from build123d import *

# Parameters (mm, degrees)
SKETCH1_W                 = 5
SKETCH1_H                 = 7
BOSS_EXTRUDE1_DEPTH       = 2
BOSS_EXTRUDE3_DEPTH       = 3
SKETCH13_W                = 5
SKETCH13_H                = 4
BOSS_EXTRUDE4_DEPTH       = 7
SKETCH14_W                = 4
SKETCH14_H                = 4
BOSS_EXTRUDE6_DEPTH       = 3
FILLET1_R                 = 2.5
M2_CLEARANCE_HOLE3_REACH  = 20.453
M2_CLEARANCE_HOLE3_BORE_R = 1.2
SKETCH15_W                = 3.5
SKETCH15_H                = 4.5
CUT_EXTRUDE1_DEPTH        = 4
M2_CLEARANCE_HOLE2_D      = 2.4
M2_CLEARANCE_HOLE2_DEPTH  = 4
M2_CLEARANCE_HOLE2_TIP    = 0.721032743
SKETCH22_W                = 4
SKETCH22_H                = 16
CUT_EXTRUDE2_DEPTH        = 3


with BuildPart() as part:
    # Sketch1 → Boss-Extrude1 (new, symmetric)
    with BuildSketch(Plane.XY):
        Rectangle(SKETCH1_W, SKETCH1_H)
    extrude(amount=BOSS_EXTRUDE1_DEPTH, both=True)

    # Sketch9 → Boss-Extrude3 (add)
    with BuildSketch(Plane.XZ.offset(3.5)):
        Polygon((2.5, 2), (6.5, 2), (6.5, -2), (2.5, -2), (-2.5, -2), (-2.5, 2), (-2.5, 14), (2.5, 14), align=None)
    extrude(amount=BOSS_EXTRUDE3_DEPTH)

    # Sketch13 → Boss-Extrude4 (add)
    with BuildSketch(Plane(origin=(0, -3.5, 0), x_dir=(1, 0, 0), z_dir=(0, 1, 0))):
        with Locations((0, -12)):
            Rectangle(SKETCH13_W, SKETCH13_H)
    extrude(amount=BOSS_EXTRUDE4_DEPTH)

    # Sketch14 → Boss-Extrude6 (add)
    with BuildSketch(Plane(origin=(0, -3.5, 0), x_dir=(1, 0, 0), z_dir=(0, 1, 0))):
        with Locations((4.5, -12)):
            Rectangle(SKETCH14_W, SKETCH14_H)
    extrude(amount=-BOSS_EXTRUDE6_DEPTH)

    # Fillet1
    # the kernel refuses this fillet: 2.5 mm, written as the material it adds along each edge
    with BuildSketch(Plane(origin=(2.5, -3.5, 2), x_dir=(0, 0, 1), z_dir=(0, -1, 0))) as fillet1_piece_1:
        with BuildLine():
            CenterArc((FILLET1_R, -FILLET1_R), FILLET1_R, 90, 90)
            Line((0, -FILLET1_R), (0, 0))
            Line((0, 0), (FILLET1_R, 0))
        make_face()
    extrude(amount=3)
    with BuildSketch(Plane(origin=(2.5, -3.5, 10), x_dir=(0, 0, -1), z_dir=(0, -1, 0))) as fillet1_piece_2:
        with BuildLine():
            CenterArc((FILLET1_R, FILLET1_R), FILLET1_R, 180, 90)
            Line((0, FILLET1_R), (0, 0))
            Line((0, 0), (FILLET1_R, 0))
        make_face()
    extrude(amount=3)

    # M2 Clearance Hole3 bore → M2 Clearance Hole3 (cut, up to next)
    with BuildSketch(Plane.XY.offset(14), mode=Mode.PRIVATE) as m2_clearance_hole3_sk1:
        Circle(M2_CLEARANCE_HOLE3_BORE_R)
    m2_clearance_hole3_tool1 = extrude(m2_clearance_hole3_sk1.sketch, amount=-M2_CLEARANCE_HOLE3_REACH, mode=Mode.PRIVATE) & part.part
    add(m2_clearance_hole3_tool1.solids().sort_by_distance((0, 0, 14))[0], mode=Mode.SUBTRACT)

    # Sketch15 → Cut-Extrude1 (cut)
    with BuildSketch(Plane(origin=(0, 0, -2), x_dir=(-1, 0, 0), z_dir=(0, 0, -1))):
        Rectangle(SKETCH15_W, SKETCH15_H)
    extrude(amount=-CUT_EXTRUDE1_DEPTH, mode=Mode.SUBTRACT)

    # M2 Clearance Hole2
    with Locations(Plane(origin=(0, -3.5, 0), x_dir=(1, 0, 0), z_dir=(0, 1, 0))):
        with Locations((4.5, -12), (0, -8), (0, -4), (4.5, 0)):
            Hole(M2_CLEARANCE_HOLE2_D / 2, depth=M2_CLEARANCE_HOLE2_DEPTH)
            with Locations((0, 0, -(M2_CLEARANCE_HOLE2_DEPTH + M2_CLEARANCE_HOLE2_TIP / 2))):  # 118° drill point
                Cone(0, M2_CLEARANCE_HOLE2_D / 2, M2_CLEARANCE_HOLE2_TIP, mode=Mode.SUBTRACT)

    # Sketch22 → Cut-Extrude2 (cut)
    with BuildSketch(Plane(origin=(0, -3.5, 0), x_dir=(1, 0, 0), z_dir=(0, 1, 0))):
        with Locations((4.5, -6)):
            Rectangle(SKETCH22_W, SKETCH22_H)
    extrude(amount=-CUT_EXTRUDE2_DEPTH, mode=Mode.SUBTRACT)


solid = part.part
The listing builds one solid part. Answer for the finished solid, in the listing's coordinates (mm). A direction names the side the tool comes from. Round coordinates to 2 decimals unless told otherwise and drop trailing zeros. Loops run counter-clockwise (first coordinate to the right, second up) from the corner with the lowest first, then second, coordinate; pieces in that order, holes last. Notation, with made-up numbers: M -21,69.5 L 22,69.5 A22 cw 22,104.5 Z; hole C 81.25,73.5 d11. An arc over 180 degrees is marked long. Write each question's results on one line, items separated by ' | '. Start each with the question number.
1) Find section D-D on z = 1.75. Write down the section's boundary in (x, y), plus the area to 4 significant figures.
2) Straight lines are drawn through the part: probe 1 along Z at (x, y) = (0, -5.2); probe 2 along Z at (x, y) = (2, -1.75); probe 3 along Y at (x, z) = (-1.05, 1). For each, find the intervals that lie inside material, in ascending order.
3) Which of the six approach directions +Z, -Z, +X, -X, +Y, -Y give full straight-line access (tool end or side, diameter ignored) to faces 1 (the flat face through (-1.75, 0, 0)), 2 (the cylindrical face through (-0.65, -5.02, 2.99)), 3 (the flat face through (0, -3.5, 6))?
4) Each of these flat-tipped pins is pushed along its axis until it touches: pin 1 (3 mm diameter, centred on x = 0, y = 0, fed in from -Z); pin 2 (1.5 mm diameter, centred on x = 0.5, z = 5.5, fed in from +Y). Where does it stop, or does it pass through?
5) Find section A-A on z = 8. Write down the section's boundary in (x, y).
6) Find section C-C on y = 1.5. Write down the section's boundary in (x, z), plus the area to 3 significant figures.
7) Find section B-B on x = -1.5. Write down the section's boundary in (y, z), plus the area to 3 significant figures.
8) Determine the mould class of faces 4 (the cylindrical face through (-0.65, -5.02, 6.99)), 5 (the flat face through (-2.5, -4, 6)), 6 (the flat face through (2, 0, 2)), 7 (the flat face through (2.5, -4, 6)) for opening direction X: pulls with the +X half, pulls with the -X half, needs draft (parallel to the pull), parting line crosses it, or undercut.
Final values:
1) outline: M -2.5,-6.5 L 2.5,-6.5 L 2.5,3.5 L -2.5,3.5 Z; hole M -1.75,-2.25 L 1.75,-2.25 L 1.75,2.25 L -1.75,2.25 Z | area: 34.25 mm²
2) probe 1: -2 to 2.8, 5.2 to 6.8, 9.2 to 14 | probe 2: -2 to 2, 10 to 14 | probe 3: -6.5 to -2.25, 2.25 to 3.5
3) face 1: -Z | face 2: +Y, -Y | face 3: +X, -X, +Y
4) pin 1: z = 10 | pin 2: y = -3.5
5) outline: M -2.5,-6.5 L -1.2,-6.5 L -1.2,-3.5 L -2.5,-3.5 Z; M 1.2,-6.5 L 2.5,-6.5 L 2.5,-3.5 L 1.2,-3.5 Z
6) outline: M -2.5,-2 L -1.75,-2 L -1.75,2 L -2.5,2 Z; M -2.5,10 L 2.5,10 L 2.5,14 L -2.5,14 Z; M 1.75,-2 L 2.5,-2 L 2.5,2 L 1.75,2 Z | area: 26.0 mm²
7) outline: M -6.5,-2 L -2.25,-2 L -2.25,2 L -3.5,2 L -3.5,10 L 3.5,10 L 3.5,14 L -6.5,14 Z; M 2.25,-2 L 3.5,-2 L 3.5,2 L 2.25,2 Z | area: 86.0 mm²
8) face 4: undercut | face 5: pulls with the -X half | face 6: needs draft | face 7: pulls with the +X half
